Study the drawing (mm; zero at the part's minimum x, y, z) and answer. A direction names the side the tool comes from. Coordinates: 2 decimals unless noted, no trailing zeros. Loops run counter-clockwise (first coordinate to the right, second up) from the corner with the lowest first, then second, coordinate; pieces in that order, holes last. Notation, with made-up numbers: (-35, 23) -> (3, 23) arc R17 cw to (3, 35) -> close; hole circle Ø7 at (-27.75, 50). An arc over 180 degrees is marked (long way). Answer as a JSON object with one key per item and string values. Group by question number.
Q1. The part is cut by section C-C on x = 8.5. Write down the section's boundary in (y, z).
Q2. The part is cut by section B-B on z = 5. Write down the section's boundary in (x, y).
Q3. Determine the mould class of the marked faces 1, 2 and 3 for opening direction X: released by +X, released by -X, zero draft, split by the parting line, or undercut.
Q4. For the marked faces 4, 5 and 6, determine the directions among +Z, -Z, +X, -X, +Y, -Y from which every point of the face is accessible in a straight line to the end or side of a thin tool.
Q5. The part is cut by section A-A on y = 30. Write down the section's boundary in (x, z).
Q6. Each of these flat-tipped pins is pushed along its axis until it touches: P1, Ø1.5, axis at x = 8, z = 5.5, coming from the +Y side; P2, Ø2.5, axis at y = 1.5, z = 4, coming from the -X side. Where does it stop, or does it pass through?
Q7. The part is cut by section D-D on z = 8.75. Write down the section's boundary in (x, y).
Q8. Straight lines are drawn through the part: line 1 along X through (y, z) = (2.1, 5); line 2 along X through (y, z) = (11, 5.5); line 3 along Z through (x, y) = (8.5, 1.1). For each, find the intervals that lie inside material, in ascending order. Write a range as [from, to].
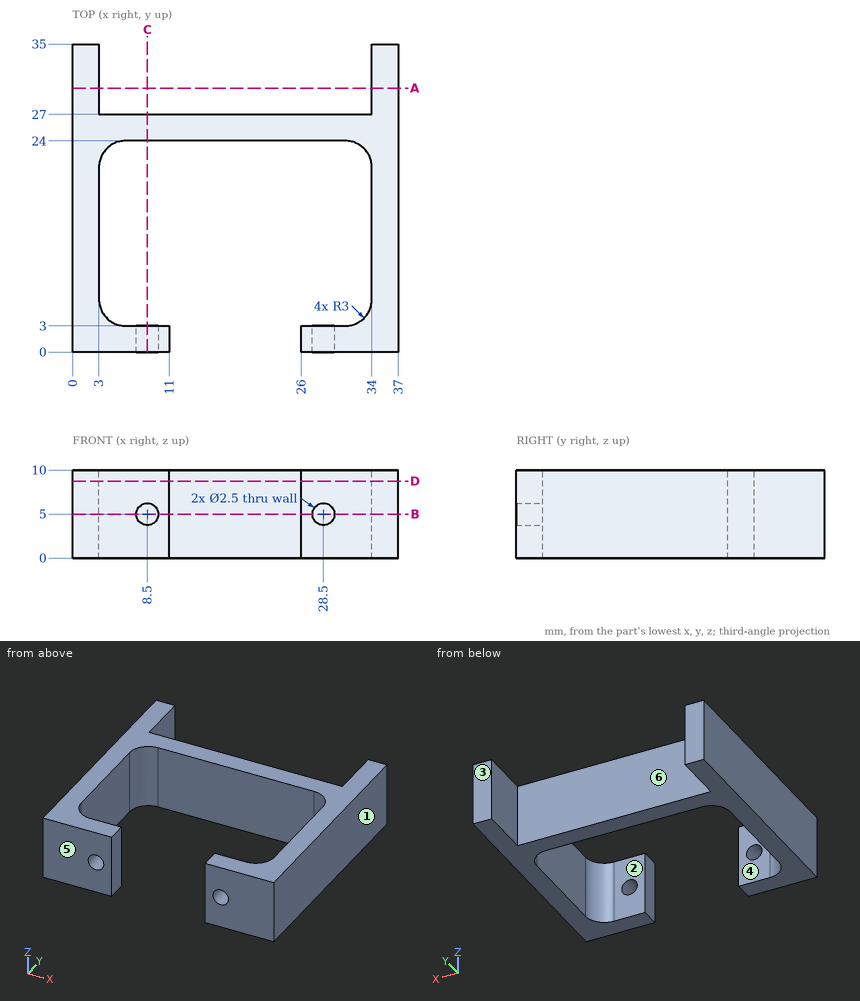
Final values:
{
 "1": {"outline": "(0, 0) -> (3, 0) -> (3, 3.75) -> (0, 3.75) -> close; (0, 6.25) -> (3, 6.25) -> (3, 10) -> (0, 10) -> close; (24, 0) -> (27, 0) -> (27, 10) -> (24, 10) -> close"},
 "2": {"outline": "(0, 0) -> (7.25, 0) -> (7.25, 3) -> (6, 3) arc R3 cw to (3, 6) -> (3, 21) arc R3 cw to (6, 24) -> (31, 24) arc R3 cw to (34, 21) -> (34, 6) arc R3 cw to (31, 3) -> (29.75, 3) -> (29.75, 0) -> (37, 0) -> (37, 35) -> (34, 35) -> (34, 27) -> (3, 27) -> (3, 35) -> (0, 35) -> close; (9.75, 0) -> (11, 0) -> (11, 3) -> (9.75, 3) -> close; (26, 0) -> (27.25, 0) -> (27.25, 3) -> (26, 3) -> close"},
 "3": {"face 1": "released by +X", "face 2": "undercut", "face 3": "zero draft"},
 "4": {"face 4": "+Z, -Z", "face 5": "+Z, -Z, +X, -X, -Y", "face 6": "+Z, -Z, +Y"},
 "5": {"outline": "(0, 0) -> (3, 0) -> (3, 10) -> (0, 10) -> close; (34, 0) -> (37, 0) -> (37, 10) -> (34, 10) -> close"},
 "6": {"P1": "stops at y = 27", "P2": "stops at x = 0"},
 "7": {"outline": "(0, 0) -> (11, 0) -> (11, 3) -> (6, 3) arc R3 cw to (3, 6) -> (3, 21) arc R3 cw to (6, 24) -> (31, 24) arc R3 cw to (34, 21) -> (34, 6) arc R3 cw to (31, 3) -> (26, 3) -> (26, 0) -> (37, 0) -> (37, 35) -> (34, 35) -> (34, 27) -> (3, 27) -> (3, 35) -> (0, 35) -> close"},
 "8": {"line 1": "x = [0, 7.25], [9.75, 11], [26, 27.25], [29.75, 37]", "line 2": "x = [0, 3], [34, 37]", "line 3": "z = [0, 3.75], [6.25, 10]"}
}
